Part model, mm, in its own coordinate system. A direction names the side the tool comes from. Give positions to 0.01 mm unless a question says otherwise; leave off trailing zeros. Order: outer loops, then holes, each group sorted by start corner. A loop starts at its lowest first (then second) coordinate and runs counter-clockwise, first axis right, second up. Notation, with made-up numbers: M 87.5,21.25 L 97.5,21.25 A15 cw 97.5,30.25 Z; hole C 12,63 d4. An arc over 180 degrees is marked long. One line per question, with ' | ' between items.
Autodesk Inventor part; units mm, degrees
ref_plane "YZ Plane" through (0, 0, 0) normal (1, 0, 0) x (0, 1, 0)
ref_plane "XZ Plane" through (0, 0, 0) normal (0, 1, 0) x (-1, 0, 0)
ref_plane "XY Plane" through (0, 0, 0) normal (0, 0, 1) x (1, 0, 0)
sketch "Sketch1" plane through (0, 0, 0) normal (0, 1, 0) x (-1, 0, 0)
  line L0 (0, 0) -> (-76.2, 0)
  line L1 (-76.2, 0) -> (-76.2, -152.4)
  line L2 (-76.2, -152.4) -> (-177.8, -152.4)
  line L3 (0, -660.4) -> (-76.2, -660.4)
  line L4 (-76.2, -660.4) -> (-76.2, -508)
  line L5 (-76.2, -508) -> (-177.8, -508)
  line L6 (0, 0) -> (0, -660.4)
  line L7 (-177.8, -152.4) -> (-177.8, -508)
  dimension "d4" = 660.4
  dimension "d91" = 152.4
  dimension "d92" = 152.4
  dimension "d95" = 177.8
  dimension "d96" = 101.6
  dimension "d97" = 101.6
  dimension "d98" = 177.8
extrude "Extrusion1" add sketch "Sketch1" along normal blind 1.5875
sketch "Sketch3" plane through (0, 1.5875, 0) normal (0, 1, 0) x (1, 0, 0)
  line L0 (0, 0) -> (76.2, 0)
  line L1 (76.2, 0) -> (76.2, 152.4)
  line L2 (76.2, 152.4) -> (177.8, 152.4)
  line L3 (177.8, 152.4) -> (177.8, 508)
  line L4 (177.8, 508) -> (76.2, 508)
  line L5 (76.2, 508) -> (76.2, 660.4)
  line L6 (76.2, 660.4) -> (0, 660.4)
  line L7 (0, 660.4) -> (0, 0)
  line L8 (1.5875, 658.8125) -> (74.6125, 658.8125)
  line L9 (74.6125, 658.8125) -> (74.6125, 506.4125)
  line L10 (74.6125, 506.4125) -> (177.8, 506.4125)
  line L11 (177.8, 153.9875) -> (74.6125, 153.9875)
  line L12 (74.6125, 153.9875) -> (74.6125, 1.5875)
  line L13 (74.6125, 1.5875) -> (1.5875, 1.5875)
  line L14 (1.5875, 1.5875) -> (1.5875, 658.8125)
  line L15 (177.8, 0) -> (179.3875, 0)
  line L16 (179.3875, 0) -> (179.3875, 660.4)
  line L17 (179.3875, 660.4) -> (177.8, 660.4)
  line L18 (177.8, 660.4) -> (177.8, 0)
  dimension "d114" = 1.5875
  dimension "d115" = 1.5875
  dimension "d116" = 1.5875
extrude "Extrusion4" add sketch "Sketch3" along normal blind 150.8125 contours L7 L6 L5 L4 L3 L10 L9 L8 L14 L13 L12 L11 L2 L1 L0
sketch "Sketch6" plane through (0, 0, -660.4) normal (-1, 0, 0) x (0, 0, 1)
  line L0 (330.2, 152.4) -> (330.2, 0) construction
  line L1 (0, 76.2) -> (660.4, 76.2) construction
  line L2 (228.6, 44.45) -> (431.8, 44.45)
  line L3 (431.8, 44.45) -> (431.8, 107.95)
  line L4 (431.8, 107.95) -> (228.6, 107.95)
  line L5 (228.6, 107.95) -> (228.6, 44.45)
  line L6 (228.6, 44.45) -> (431.8, 107.95) construction
  line L7 (431.8, 44.45) -> (228.6, 107.95) construction
  line L8 (190.5, 44.45) -> (114.3, 44.45)
  line L9 (114.3, 44.45) -> (114.3, 107.95)
  line L10 (114.3, 107.95) -> (190.5, 107.95)
  line L11 (190.5, 107.95) -> (190.5, 44.45)
  line L12 (190.5, 44.45) -> (114.3, 107.95) construction
  line L13 (114.3, 44.45) -> (190.5, 107.95) construction
  line L14 (469.9, 44.45) -> (546.1, 44.45)
  line L15 (546.1, 44.45) -> (546.1, 107.95)
  line L16 (546.1, 107.95) -> (469.9, 107.95)
  line L17 (469.9, 107.95) -> (469.9, 44.45)
  line L18 (469.9, 44.45) -> (546.1, 107.95) construction
  line L19 (546.1, 44.45) -> (469.9, 107.95) construction
  line L20 (0, 152.4) -> (660.4, 152.4)
  line L21 (0, 0) -> (0, 152.4)
  point P0 (330.2, 76.2)
  point P1 (152.4, 76.2)
  point P2 (508, 76.2)
  dimension "d21" = 203.2
  dimension "d22" = 63.5
  dimension "d23" = 76.2
  dimension "d24" = 63.5
  dimension "d25" = 38.1
  dimension "d26" = 76.2
  dimension "d27" = 63.5
  dimension "d28" = 38.1
extrude "Extrusion6" add sketch "Sketch3" along normal blind 150.8125 and the other way blind 1.5875 contours L3 L18 L17 L16 L15
extrude "Extrusion7" cut sketch "Sketch6" against normal up to surface (1.5875 mm away)
sketch "Sketch8" plane through (179.3875, 0, -660.4) normal (1, 0, 0) x (0, 0, -1)
  circle A0 centre (-584.2, 76.2) radius 14.2875
  circle A1 centre (-76.2, 76.2) radius 14.2875
  line L0 (-660.4, 152.4) -> (0, 152.4)
  line L1 (-660.4, 0) -> (-660.4, 152.4)
  line L2 (0, 0) -> (0, 152.4)
  dimension "d117" = 28.575
  dimension "d118" = 28.575
  dimension "d119" = 76.2
  dimension "d120" = 76.2
  dimension "d121" = 76.2
  dimension "d122" = 76.2
extrude "Extrusion9" cut sketch "Sketch8" against normal up to surface (104.775 mm away)
equation "\"d96\" = d97"
equation "\"d98\" = d95"
equation "\"d24\" = d22"
equation "\"d27\" = d22"
equation "\"d28\" = d25"
properties part number "DriveHousing" material "Aluminum 6061"
1. Slice it at B-B on z = -138.5. Give the cut face in (x, y).
Worked out:
outline: M 0,0 L 76.2,0 L 76.2,152.4 L 74.61,152.4 L 74.61,1.59 L 1.59,1.59 L 1.59,44.45 L 0,44.45 Z; M 0,107.95 L 1.59,107.95 L 1.59,152.4 L 0,152.4 Z; M 177.8,0 L 179.39,0 L 179.39,152.4 L 177.8,152.4 Z
2. Slice it at C-C on y = 33. Give the cut face in (x, z), then the cut area to 3 significant figures.
Worked out:
outline: M 0,-660.4 L 76.2,-660.4 L 76.2,-508 L 177.8,-508 L 177.8,-660.4 L 179.39,-660.4 L 179.39,0 L 177.8,0 L 177.8,-152.4 L 76.2,-152.4 L 76.2,0 L 0,0 Z; hole M 1.59,-658.81 L 74.61,-658.81 L 74.61,-506.41 L 177.8,-506.41 L 177.8,-153.99 L 74.61,-153.99 L 74.61,-1.59 L 1.59,-1.59 Z | area: 3,140 mm2
3. Slice it at A-A on z = -270. Give the cut face in (x, y).
Worked out:
outline: M 0,0 L 179.39,0 L 179.39,152.4 L 177.8,152.4 L 177.8,1.59 L 1.59,1.59 L 1.59,44.45 L 0,44.45 Z; M 0,107.95 L 1.59,107.95 L 1.59,152.4 L 0,152.4 Z
4. Probe L1, parallel to X at y = 67.5, z = -550; L2, parallel to Z at x = 112, y = 93; L3, parallel to Z at x = 178, y = 76. List the from-to ranges inside material, lowest first. Write a range as from..to.
Worked out:
L1: x = 0..1.59, 74.61..76.2, 177.8..179.39 | L2: z = -508..-506.41, -153.99..-152.4 | L3: z = -660.4..-598.49, -569.91..-90.49, -61.91..0
5. Slice it at D-D on x = 115. Give the cut face in (y, z).
Worked out:
outline: M 0,-508 L 152.4,-508 L 152.4,-506.41 L 1.59,-506.41 L 1.59,-153.99 L 152.4,-153.99 L 152.4,-152.4 L 0,-152.4 Z
6. Drop flat-ended pins along their axis: pin 1 (4 mm diameter, centred on y = 62, z = -125.5, fed in from -X); pin 2 (1 mm diameter, centred on x = 97.5, z = -180, fed in from +Y). Give the stop position or say it passes through.
Worked out:
pin 1: stops at x = 74.61 | pin 2: stops at y = 1.59
7. Tool access for faces 4 (the flat face through (74.612, 93, -584)), 5 (the flat face through (177.8, 75, -566)), 6 (the flat face through (69, 0, -335)), 7 (the flat face through (177.8, 92, -75)), 8 (the cylindrical face through (178.605, 90.366, -74.34)): list every direction of +Z, -Z, +X, -X, +Y, -Y with a clear straight run to the whole face (end or side of a thin tool).
Worked out:
face 4: +Y | face 5: -Z, +Y, -Y | face 6: +Z, -Z, +X, -X, -Y | face 7: +Z, +Y, -Y | face 8: +X
8. Mould opens along X. For faces 1 (the flat face through (179.388, 75, -326)), 2 (the cylindrical face through (75.417, 90.366, -74.34)), 3 (the flat face through (127, 76, -153.988)) say: released by +X, released by -X, zero draft, split by the parting line, or undercut.
Worked out:
face 1: released by +X | face 2: zero draft | face 3: undercut
